```python
from build123d import *

# Parameters (mm, degrees)
F0_W     = 50.8
F0_H     = 50.8
F1_DEPTH = 50.8
F2_W     = 38.1
F2_H     = 38.1
F3_DEPTH = 50.801
F4_W     = 25.4
F4_H     = 25.4
F5_DEPTH = 50.801


with BuildPart() as f1:
    # F0 (on Front) → F1 (new body)
    with BuildSketch(Plane.XZ):
        with Locations((-73.563374, 19.488397)):
            Rectangle(F0_W, F0_H)
    extrude(amount=F1_DEPTH)

    # F2 (on face) → F3 (cut, through all)
    with BuildSketch(Plane.XZ.offset(50.8)):
        with Locations((-73.563374, 19.488397)):
            Rectangle(F2_W, F2_H)
    extrude(amount=-F3_DEPTH, mode=Mode.SUBTRACT)

    # F4 (on face) → F5 (cut, through all)
    with BuildSketch(Plane.XY.offset(44.888397)):
        with Locations((-73.563374, -25.4)):
            Rectangle(F4_W, F4_H)
    extrude(amount=-F5_DEPTH, mode=Mode.SUBTRACT)


solid = f1.part
```
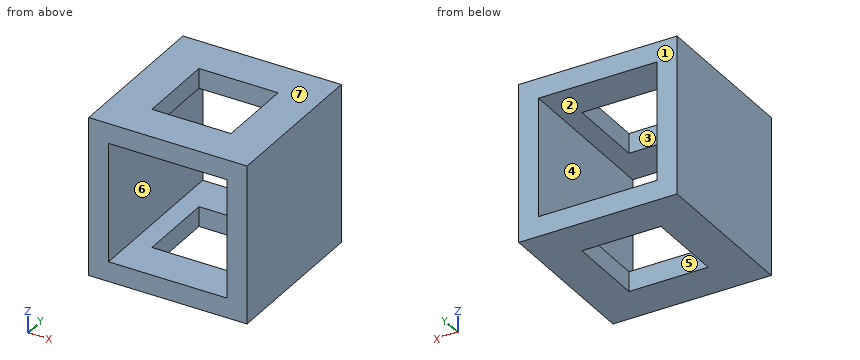
CAD build for the part. Positions are in the model's coordinates, mm. Face numbers are marked on the shaded views. A direction names the side the tool comes from. Round coordinates to 2 decimals unless told otherwise and drop trailing zeros. Order: outer loops, then holes, each group sorted by start corner. A loop starts at its lowest first (then second) coordinate and runs counter-clockwise, first axis right, second up.
Q1. Slice it at C-C (z = 28). Write the cut outline in (x, y), and give its area (3 significant figures).
Q2. Wall check: L1, parallel to X at y = -44.5, z = 30.5; L2, parallel to Z at x = -60, y = -25.5; L3, parallel to Y at x = -82, z = -0.5. Give the ranges that are in metal, low to high.
Q3. Which spindle directions (+Z, -Z, +X, -X, +Y, -Y) get a long thin tool onto all of the face, cutting with end or side? Do the marked faces 1, 2 and 3. Say none if no direction does.
Q4. Slice it at D-D (y = -45). Write the cut outline in (x, z), and give its area (3 significant figures).
Q5. Slice it at B-B (x = -65.5). Write the cut outline in (y, z), and give its area (3 significant figures).
Q6. Slice it at A-A (y = -26.5). Write the cut outline in (x, z).
Q7. Two-plate mould, pull along Z, no slides. Class the marked faces 4, 5, 6 and 7: pulls with the +Z half, pulls with the -Z half, needs draft (parallel to the pull), parting line crosses it, or undercut.
Results below:
1. outline: (-98.96, -50.8) - (-92.61, -50.8) - (-92.61, 0) - (-98.96, 0) - close; (-54.51, -50.8) - (-48.16, -50.8) - (-48.16, 0) - (-54.51, 0) - close
1. area: 645 mm2
2. L1: x = -98.96 to -92.61, -54.51 to -48.16
2. L2: z = -5.91 to 0.44, 38.54 to 44.89
2. L3: y = -50.8 to -38.1, -12.7 to 0
3. face 1: +Z, -Z, +X, -X, +Y
3. face 2: +Y, -Y
3. face 3: +Z, -Z
4. outline: (-98.96, -5.91) - (-48.16, -5.91) - (-48.16, 44.89) - (-98.96, 44.89) - close; hole (-92.61, 0.44) - (-54.51, 0.44) - (-54.51, 38.54) - (-92.61, 38.54) - close
4. area: 1,130 mm2
5. outline: (-50.8, -5.91) - (-38.1, -5.91) - (-38.1, 0.44) - (-50.8, 0.44) - close; (-50.8, 38.54) - (-38.1, 38.54) - (-38.1, 44.89) - (-50.8, 44.89) - close; (-12.7, -5.91) - (0, -5.91) - (0, 0.44) - (-12.7, 0.44) - close; (-12.7, 38.54) - (0, 38.54) - (0, 44.89) - (-12.7, 44.89) - close
5. area: 323 mm2
6. outline: (-98.96, -5.91) - (-86.26, -5.91) - (-86.26, 0.44) - (-92.61, 0.44) - (-92.61, 38.54) - (-86.26, 38.54) - (-86.26, 44.89) - (-98.96, 44.89) - close; (-60.86, -5.91) - (-48.16, -5.91) - (-48.16, 44.89) - (-60.86, 44.89) - (-60.86, 38.54) - (-54.51, 38.54) - (-54.51, 0.44) - (-60.86, 0.44) - close
7. face 4: undercut
7. face 5: needs draft
7. face 6: undercut
7. face 7: pulls with the +Z half
